Here's how the part is built. I have some questions about the finished solid (model axes, mm). A direction names the side the tool comes from. Coordinates: 2 decimals unless noted, no trailing zeros. Write each loop counter-clockwise with the first axis right and the second up, starting at its lowest first coordinate (ties: lowest second). Pieces come first, ordered by that corner, then holes.
(1) For pin 1 Ø11 at (x, y) = (419.45, 105) entering from +Z, with a flat end and sliding along its axis, tell me the tip position at first contact or that it passes through.
(2) Please list where these lines run through material, in increasing order: probe 1 along Y at (x, z) = (477.5, 0.6); probe 2 along X at (y, z) = (29.5, 0.3); probe 3 along Y at (x, z) = (460, -1.3).
(3) Imagine slicing it at C-C, the plane x = 451. List the corners of the cut face in (y, z) for me, plus the area to 3 significant figures.
(4) Imagine slicing it at B-B, the plane y = 53.5. List the corners of the cut face in (x, z) for me, plus the area to 4 significant figures.
(5) Imagine slicing it at A-A, the plane x = 462. List the corners of the cut face in (y, z) for me, plus the area to 3 significant figures.
(6) Imagine slicing it at D-D, the plane z = -0.6. State how many separate pieces and enclosed holes the cut face has, plus the area to 3 significant figures.
(7) Thinking about a two-plate mould opening in Y: for faces 1 (the flat face through (425.417, 121, 0)), 2 (the flat face through (451, 152, 0)), 3 (the flat face through (451, -2, 0)), 4 (the flat face through (410.417, 74, 0)), which applies, released by +Y, released by -Y, zero draft, split by the parting line, or undercut?
(8) Which directions (+Z, -Z, +X, -X, +Y, -Y) give clear straight access to the entire face, cutting with the end or side of a thin tool? Please do faces 5 (the flat face through (481, 30.647, 0)), 6 (the flat face through (492.916, 75, 0)).
```python
from build123d import *

# Parameters (mm, degrees)
SALIENTE_EXTRUIR1_START = -1.5
SALIENTE_EXTRUIR1_DEPTH = 3
CROQUIS4_W              = 30
CROQUIS4_H              = 60
CORTAR_EXTRUIR3_DEPTH   = 10
CROQUIS5_W              = 9.999999994
CROQUIS5_H              = 3
CROQUIS5_W_2            = 9.587122789
CORTAR_EXTRUIR4_DEPTH   = 10
CROQUIS6_R              = 1.9
CORTAR_EXTRUIR5_DEPTH   = 10
REDONDEO1_R             = 5
CROQUIS7_W              = 82.5
CROQUIS7_H              = 3
SALIENTE_EXTRUIR2_DEPTH = 2
CROQUIS8_W              = 82.49989544
CROQUIS8_H              = 3
SALIENTE_EXTRUIR3_DEPTH = 2
CROQUIS9_R              = 4.181897372
CORTAR_EXTRUIR6_DEPTH   = 10


# Read off the part's stored shape, not the designer's step: Saliente-Extruir1
with BuildPart() as part:
    # Saliente-Extruir1 outline → Saliente-Extruir1 (new body)
    with BuildSketch(Plane.XY.offset(SALIENTE_EXTRUIR1_START)):
        with BuildLine():
            ThreePointArc((492.916449572, 98.009593947), (492.452410006, 99.442022929), (491.249851225, 100.348134338))
            ThreePointArc((491.249851225, 100.348134338), (487.916517891, 105.062179546), (491.249851225, 109.776224754))
            ThreePointArc((491.249851225, 109.776224754), (492.452037009, 110.681812922), (492.916439741, 112.113480025))
            Line((492.916439741, 112.113480025), (492.916413331, 149.999679341))
            Line((492.916413331, 149.999679341), (410.416517891, 149.999679341))
            Line((410.416517891, 149.999679341), (410.416517891, -0.000320659))
            Line((410.416517891, -0.000320659), (492.916517891, -0.000320659))
            Line((492.916517891, -0.000320659), (492.916491488, 37.877716604))
            ThreePointArc((492.916491488, 37.877716604), (492.45443711, 39.314289338), (491.249851225, 40.223249354))
            ThreePointArc((491.249851225, 40.223249354), (487.916517891, 44.937294562), (491.249851225, 49.65133977))
            ThreePointArc((491.249851225, 49.65133977), (492.453865854, 50.559496169), (492.916481647, 51.994900607))
            Line((492.916481647, 51.994900607), (492.916449572, 98.009593947))
        make_face()
    extrude(amount=SALIENTE_EXTRUIR1_DEPTH)

    # Croquis4 → Cortar-Extruir3 (cut)
    with BuildSketch(Plane.XY.offset(1.5)):
        with Locations((455.222459901, 75.336681949)):
            Rectangle(CROQUIS4_W, CROQUIS4_H)
    extrude(amount=-CORTAR_EXTRUIR3_DEPTH, mode=Mode.SUBTRACT)

    # Croquis5 → Cortar-Extruir4 (cut)
    with BuildSketch(Plane(origin=(0, 0, -1.5), x_dir=(-1, 0, 0), z_dir=(0, 0, -1))):
        with Locations((-420.82939509, 29.146675475)):
            Rectangle(CROQUIS5_W, CROQUIS5_H)
        with Locations((-480.921167725, 29.146675475)):
            Rectangle(CROQUIS5_W, CROQUIS5_H)
        with Locations((-480.921167725, 120.852683208)):
            Rectangle(CROQUIS5_W, CROQUIS5_H)
        with Locations((-420.622956488, 120.852683208)):
            Rectangle(CROQUIS5_W_2, CROQUIS5_H)
    extrude(amount=-CORTAR_EXTRUIR4_DEPTH, mode=Mode.SUBTRACT)

    # Croquis6 → Cortar-Extruir5 (cut)
    with BuildSketch(Plane.XY.offset(1.5)):
        with Locations((450.875281407, 29.146675475)):
            Circle(CROQUIS6_R)
        with Locations((450.875281407, 120.857819079)):
            Circle(CROQUIS6_R)
    extrude(amount=-CORTAR_EXTRUIR5_DEPTH, mode=Mode.SUBTRACT)

    # Redondeo1
    redondeo1_edges = [part.edges().sort_by_distance(p)[0] for p in [
        (470.222459901, 105.336681949, 0),
        (470.222459901, 45.336681949, 0),
        (440.222459901, 45.336681949, 0),
        (440.222459901, 105.336681949, 0),
    ]]
    fillet(redondeo1_edges, radius=REDONDEO1_R)

    # Croquis7 → Saliente-Extruir2 (add)
    with BuildSketch(Plane.XZ.offset(0.000320659)):
        with Locations((451.666517891, 0)):
            Rectangle(CROQUIS7_W, CROQUIS7_H)
    extrude(amount=SALIENTE_EXTRUIR2_DEPTH)

    # Croquis8 → Saliente-Extruir3 (add)
    with BuildSketch(Plane(origin=(0, 149.999679341, 0), x_dir=(1, 0, 0), z_dir=(0, 1, 0))):
        with Locations((451.666465611, 0)):
            Rectangle(CROQUIS8_W, CROQUIS8_H)
    extrude(amount=SALIENTE_EXTRUIR3_DEPTH)

    # Croquis9 → Cortar-Extruir6 (cut)
    with BuildSketch(Plane(origin=(0, 0, -1.5), x_dir=(-1, 0, 0), z_dir=(0, 0, -1))):
        with Locations((-419.456517891, 44.999679341)):
            Circle(CROQUIS9_R)
        with Locations(Location((-419.454650283, 105.000242051, 0), (0, 0, 180))):
            Circle(CROQUIS9_R)
    extrude(amount=-CORTAR_EXTRUIR6_DEPTH, mode=Mode.SUBTRACT)


solid = part.part
```
Recorded:
1. pin 1: stops at z = 1.5
2. probe 1: y = -2 to 27.65, 30.65 to 119.35, 122.35 to 152
2. probe 2: x = 410.42 to 415.83, 425.83 to 449.01, 452.74 to 475.92, 485.92 to 492.92
2. probe 3: y = -2 to 45.34, 105.34 to 152
3. outline: (-2, -1.5) - (27.25, -1.5) - (27.25, 1.5) - (-2, 1.5) - close; (31.04, -1.5) - (45.34, -1.5) - (45.34, 1.5) - (31.04, 1.5) - close; (105.34, -1.5) - (118.96, -1.5) - (118.96, 1.5) - (105.34, 1.5) - close; (122.75, -1.5) - (152, -1.5) - (152, 1.5) - (122.75, 1.5) - close
3. area: 259 mm2
4. outline: (410.42, -1.5) - (440.22, -1.5) - (440.22, 1.5) - (410.42, 1.5) - close; (470.22, -1.5) - (492.92, -1.5) - (492.92, 1.5) - (470.22, 1.5) - close
4. area: 157.5 mm2
5. outline: (-2, -1.5) - (45.34, -1.5) - (45.34, 1.5) - (-2, 1.5) - close; (105.34, -1.5) - (152, -1.5) - (152, 1.5) - (105.34, 1.5) - close
5. area: 282 mm2
6. separate pieces: 1
6. enclosed holes: 9
6. area: 10,600 mm2
7. face 1: undercut
7. face 2: released by +Y
7. face 3: released by -Y
7. face 4: zero draft
8. face 5: +Z, -Z
8. face 6: +Z, -Z, +X, +Y, -Y
